Here's how the part is built. I have some questions about the finished solid (model axes, mm). Face numbers are marked on the shaded views. Give positions to 0.01 mm unless a question says otherwise; leave off trailing zeros. Loops run counter-clockwise (first coordinate to the right, second up) from the corner with the lowest first, then second, coordinate; pieces in that order, holes last.
Q1. I need wall thicknesses on line 1 (Z direction, x = 40, y = 13.5); line 2 (X direction, y = 12.5, z = 9.5); line 3 (X direction, y = 5, z = 5.25). Which ranges of each line are inside material? Lowest first, please.
Q2. If we section it at D-D (x = 17.5): Please give me the cut outline in (y, z).
Q3. We'd pull the mould along Y, two halves only. Please class the marked faces 1, 2 and 3: +Y half, -Y half, draft (parallel to the pull), parting line (faces both ways), or undercut.
Q4. If we section it at B-B (x = 26.5): Please give me the cut outline in (y, z).
Q5. Will these pins go through, and if not, where does the flat tip stop? P1, Ø1.1, axis at y = 19, z = 9, coming from the -X side; P2, Ø1.8, axis at x = 29, z = 9, coming from the -Y side; P3, Ø6, axis at y = 8, z = 6.5, coming from the -X side.
Q6. If we section it at A-A (y = 8): Please give me the cut outline in (x, z).
Q7. If we section it at C-C (y = 12): Please give me the cut outline in (x, z).
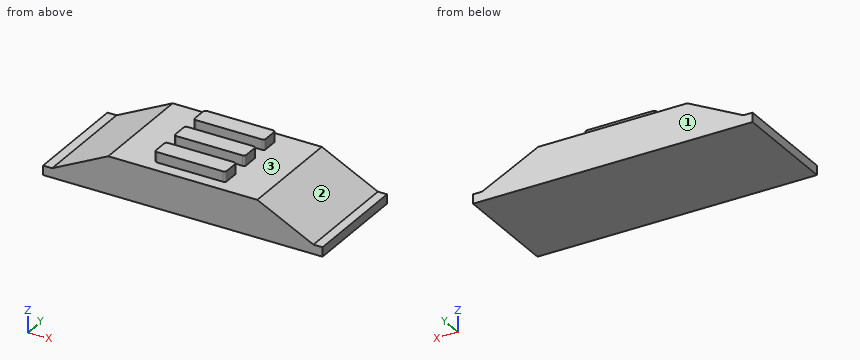
from build123d import *

# Parameters (mm, degrees)
F0_W     = 60
F0_H     = 23.2
F1_DEPTH = 2
F3_DEPTH = 23.2
F4_W     = 15.2
F4_H     = 4
F5_DEPTH = 2.2
F6_R     = 0.5


with BuildPart() as f1:
    # F0 (on Top) → F1 (new body)
    with BuildSketch(Plane.XY):
        with Locations((30, 11.6)):
            Rectangle(F0_W, F0_H)
    extrude(amount=F1_DEPTH)

    # F2 (on face) → F3 (join, through all)
    with BuildSketch(Plane(origin=(0, 23.2, 0), x_dir=(-1, 0, 0), z_dir=(0, 1, 0))):
        Polygon((-1.952949, 2), (-14, 8), (-46, 8), (-58.047051, 2), align=None)
    extrude(amount=-F3_DEPTH)

    # F4 (on face) → F5 (join)
    with BuildSketch(Plane.XY.offset(8)):
        with Locations((30, 18.6)):
            Rectangle(F4_W, F4_H)
        Polygon((22.4, 13.6), (22.4, 11.6), (22.4, 9.6), (37.6, 9.6), (37.6, 11.6), (37.6, 13.6), align=None)
        with Locations((30, 4.6)):
            Rectangle(F4_W, F4_H)
    extrude(amount=F5_DEPTH)

    # F6
    f6_edges = [f1.edges().sort_by_distance(p)[0] for p in [
        (22.4, 16.6, 9.1),
        (22.4, 9.6, 9.1),
        (22.4, 2.6, 9.1),
        (37.6, 2.6, 9.1),
        (37.6, 9.6, 9.1),
        (37.6, 16.6, 9.1),
        (22.4, 6.6, 9.1),
        (37.6, 6.6, 9.1),
        (37.6, 13.6, 9.1),
        (22.4, 13.6, 9.1),
        (22.4, 20.6, 9.1),
        (37.6, 20.6, 9.1),
    ]]
    fillet(f6_edges, radius=F6_R)


solid = f1.part
Check sheet entries:
1. line 1: z = 0 to 8
1. line 2: x = 22.4 to 37.6
1. line 3: x = 8.48 to 51.52
2. outline: (0, 0) - (23.2, 0) - (23.2, 8) - (0, 8) - close
3. face 1: +Y half
3. face 2: draft
3. face 3: undercut
4. outline: (0, 0) - (23.2, 0) - (23.2, 8) - (20.6, 8) - (20.6, 10.2) - (16.6, 10.2) - (16.6, 8) - (13.6, 8) - (13.6, 10.2) - (9.6, 10.2) - (9.6, 8) - (6.6, 8) - (6.6, 10.2) - (2.6, 10.2) - (2.6, 8) - (0, 8) - close
5. P1: stops at x = 22.4
5. P2: stops at y = 2.6
5. P3: stops at x = 4.96
6. outline: (0, 0) - (60, 0) - (60, 2) - (58.05, 2) - (46, 8) - (14, 8) - (1.95, 2) - (0, 2) - close
7. outline: (0, 0) - (60, 0) - (60, 2) - (58.05, 2) - (46, 8) - (37.6, 8) - (37.6, 10.2) - (22.4, 10.2) - (22.4, 8) - (14, 8) - (1.95, 2) - (0, 2) - close
